Read the model definition and answer for the solid it produces. Units are mm, in the model's axes. A direction names the side the tool comes from. Round coordinates to 2 decimals unless told otherwise and drop trailing zeros. Order: outer loops, then holes, each group sorted by start corner. A loop starts at its lowest first (then second) coordinate and runs counter-clockwise, first axis right, second up.
from build123d import *

# Parameters (mm, degrees)
BOSS_EXTRUDE1_DEPTH = 23
BOSS_EXTRUDE2_DEPTH = 2
SKETCH3_R           = 1.05
BOSS_EXTRUDE3_DEPTH = 14.5
SKETCH4_W           = 17
SKETCH4_H           = 23.2
CUT_EXTRUDE1_DEPTH  = 50
SKETCH7_W           = 18
SKETCH7_H           = 32
CUT_EXTRUDE4_DEPTH  = 61.367623773
SKETCH8_R           = 2
CUT_EXTRUDE5_DEPTH  = 1.4
FILLET1_R           = 2


with BuildPart() as part:
    # Sketch1 → Boss-Extrude1 (new, symmetric)
    with BuildSketch(Plane.XY):
        with BuildLine():
            Line((0, 41.7), (16.889174661, 31.949030463))
            ThreePointArc((16.889174661, 31.949030463), (17.524957173, 11.599404984), (0, 1.23661807))
            Line((0, 1.23661807), (0, 0))
            Line((0, 0), (8.83210354, 0))
            ThreePointArc((8.83210354, 0), (22.981624329, 20.31741016), (10.5, 41.7))
            Line((10.5, 41.7), (0, 41.7))
        make_face()
    extrude(amount=BOSS_EXTRUDE1_DEPTH, both=True)

    # Sketch2 → Boss-Extrude2 (add)
    with BuildSketch(Plane.XY.offset(23)):
        with BuildLine():
            Line((0, 41.7), (16.889174661, 31.949030463))
            ThreePointArc((16.889174661, 31.949030463), (17.524957173, 11.599404984), (0, 1.23661807))
            Line((0, 1.23661807), (0, 41.7))
        make_face()
    boss_extrude2 = extrude(amount=-BOSS_EXTRUDE2_DEPTH)

    # Mirror2: Boss-Extrude2 across plane
    add(boss_extrude2.mirror(Plane.XY))

    # Sketch3 → Boss-Extrude3 (add, symmetric)
    with BuildSketch(Plane.XY):
        with BuildLine():
            Line((12.5, -53), (6.5, -53))
            Line((6.5, -53), (6.5, -48))
            Line((6.5, -48), (12.5, -48))
            Line((12.5, -48), (12.5, -14))
            Line((12.5, -14), (6.5, -14))
            Line((6.5, -14), (6.5, -9))
            Line((6.5, -9), (12.5, -9))
            Line((12.5, -9), (12.5, 0))
            Line((12.5, 0), (8.83210354, 0))
            ThreePointArc((8.83210354, 0), (13.539004564, 2.643733533), (17.5, 6.311806514))
            Line((17.5, 6.311806514), (17.5, -53))
            Line((17.5, -53), (12.5, -53))
        make_face()
        with Locations(Location((9, -11.5, 0), (0, 0, 180))):
            Circle(SKETCH3_R, mode=Mode.SUBTRACT)
        with Locations(Location((9, -50.5, 0), (0, 0, 180))):
            Circle(SKETCH3_R, mode=Mode.SUBTRACT)
    extrude(amount=BOSS_EXTRUDE3_DEPTH, both=True)

    # Sketch4 → Cut-Extrude1 (cut)
    with BuildSketch(Plane.XZ.offset(53)):
        with Locations((4, 0)):
            Rectangle(SKETCH4_W, SKETCH4_H)
    extrude(amount=-CUT_EXTRUDE1_DEPTH, mode=Mode.SUBTRACT)

    # Sketch7 → Cut-Extrude4 (cut, through all)
    with BuildSketch(Plane(origin=(17.5, 0, 0), x_dir=(0, 0, -1), z_dir=(1, 0, 0))):
        with Locations((0, -31.5)):
            Rectangle(SKETCH7_W, SKETCH7_H)
    extrude(amount=-CUT_EXTRUDE4_DEPTH, mode=Mode.SUBTRACT)

    # Sketch8 → Cut-Extrude5 (cut)
    with BuildSketch(Plane.XY.offset(14.5)):
        with Locations((9, -11.5)):
            Circle(SKETCH8_R)
        with Locations((9, -50.5)):
            Circle(SKETCH8_R)
    cut_extrude5 = extrude(amount=-CUT_EXTRUDE5_DEPTH, mode=Mode.SUBTRACT)

    # Fillet1
    fillet1_edges = [part.edges().sort_by_distance(p)[0] for p in [
        (15, -15.5, -9),
        (15, -47.5, -9),
        (15, -47.5, 9),
        (15, -15.5, 9),
        (17.5, -53, 0),
        (6.5, -9, 13.05),
        (6.5, -14, 13.05),
        (6.5, -48, 13.05),
        (6.5, -53, 13.05),
        (6.5, -53, -13.05),
        (6.5, -48, -13.05),
        (6.5, -14, -13.05),
        (6.5, -9, -13.05),
    ]]
    fillet(fillet1_edges, radius=FILLET1_R)

    # Mirror3: Cut-Extrude5 across plane
    add(cut_extrude5.mirror(Plane.XY), mode=Mode.SUBTRACT)


solid = part.part
Q1. A cutting plane is placed at C-C, the plane x = 3.5. Give the vertices of the cut face in (y, z).
Outcome:
outline: (0, -23) - (41.7, -23) - (41.7, 23) - (0, 23) - close; hole (1.55, -21) - (39.68, -21) - (39.68, 21) - (1.55, 21) - close
Q2. For faces 4 (the face through (9.9, -12.4, 13.1)), 5 (the face through (14.96, -46.93, 8.4)), 6 (the face through (7.1, -13.43, -13.07)), determine the directions among +Z, -Z, +X, -X, +Y, -Y from which every point of the face is accessible in a straight line to the end or side of a thin tool.
Outcome:
face 4: +Z
face 5: +X, -X
face 6: +Z, -Z, -X
Q3. A cutting plane is placed at B-B, the plane z = -4. Give the vertices of the cut face in (x, y).
Outcome:
outline: (0, 0) - (12.5, 0) - (12.5, -15.5) - (17.5, -15.5) - (17.5, 6.31) arc R23 ccw to (10.5, 41.7) - (0, 41.7) - (16.89, 31.95) arc R20 cw to (0, 1.24) - close; (12.5, -53) - (15.5, -53) arc R2 ccw to (17.5, -51) - (17.5, -47.5) - (12.5, -47.5) - close
Q4. A cutting plane is placed at A-A, the plane y = -21. Give the vertices of the cut face in (x, z).
Outcome:
outline: (12.5, -14.5) - (17.5, -14.5) - (17.5, -9) - (12.5, -9) - close; (12.5, 9) - (17.5, 9) - (17.5, 14.5) - (12.5, 14.5) - close
Q5. Straight lines are drawn through the part: probe 1 along Z at (x, y) = (4, 20.5); probe 2 along Y at (x, z) = (9, -12.1); probe 3 along Z at (x, y) = (17.25, -29). For each, find the intervals that lie inside material, in ascending order.
Outcome:
probe 1: z = -23 to -21, 21 to 23
probe 2: y = -53 to -51.55, -49.45 to -48, -14 to -12.55, -10.45 to -9, 0 to 3.38, 36.5 to 41.7
probe 3: z = -14.5 to -9, 9 to 14.5
Q6. A cutting plane is placed at D-D, the plane y = 14.5. Give the vertices of the cut face in (x, z).
Outcome:
outline: (0, -23) - (21.99, -23) - (21.99, 23) - (0, 23) - (0, 21) - (18.83, 21) - (18.83, -21) - (0, -21) - close
Q7. Flat-ended cylindrical pins translate along their axes: pin 1 (2.5 mm diameter, centred on x = 9.5, y = -49.5, fed in from -Z); pin 2 (5.5 mm diameter, centred on x = 15, z = 2, fed in from +Y); pin 3 (1 mm diameter, centred on y = 22, z = -4, fed in from -X). Find the tip coordinate at first contact, or state that the pin passes through.
Outcome:
pin 1: stops at z = -14.5
pin 2: stops at y = 40.7
pin 3: stops at x = 19.96
Q8. For a pull along X with two mould halves and no side action, classify faces 1 (the face through (8.33, 36.89, 0.29)), 2 (the face through (9.9, -12.4, -13.1)), 3 (the face through (10.1, -11, -11.6)) as released by +X, released by -X, zero draft, split by the parting line, or undercut.
Outcome:
face 1: released by -X
face 2: undercut
face 3: zero draft
